Drawing for the job (mm, zero at the part's lowest x, y, z). Coordinates: 2 decimals unless noted, no trailing zeros. Loops run counter-clockwise (first coordinate to the right, second up) from the corner with the lowest first, then second, coordinate; pieces in that order, holes last. Notation, with made-up numbers: (31, -19.5) -> (40, -19.5) arc R26 ccw to (40, 8.5) -> close; hole circle Ø4 at (-22, 87). An arc over 180 degrees is marked (long way). Write each question's results on one line, items separated by ' | '.
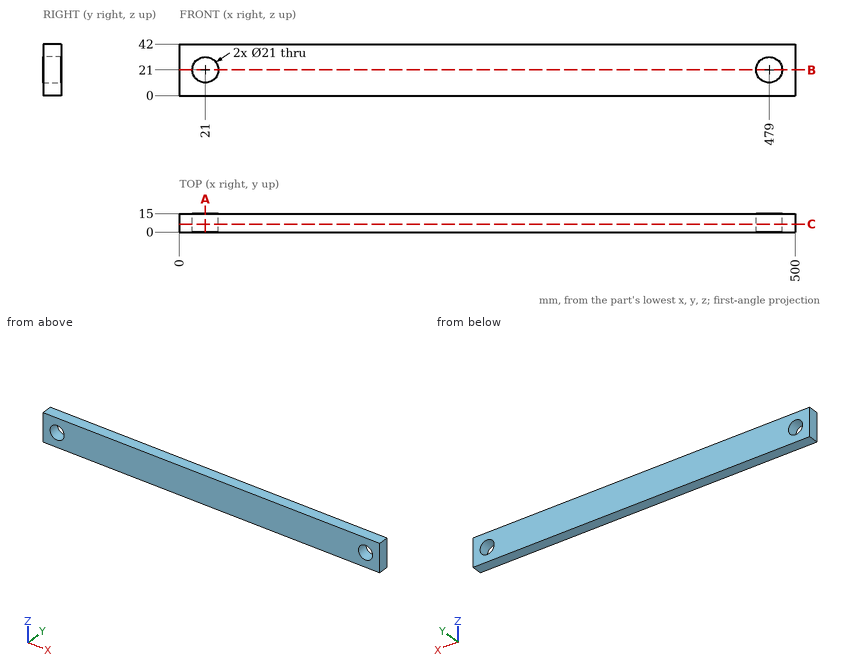
1) Drill centre lines: L1, parallel to X at y = 6.5, z = 23; L2, parallel to Z at x = 479, y = 6.5; L3, parallel to X at y = 4, z = 21. Where is each one in solid material? Low to high. Write a range as from..to.
Outcome:
L1: x = 0..10.69, 31.31..468.69, 489.31..500 | L2: z = 0..10.5, 31.5..42 | L3: x = 0..10.5, 31.5..468.5, 489.5..500
2) Slice it at A-A (x = 21). Write the cut outline in (y, z), then the cut area to 3 significant figures.
Outcome:
outline: (0, 0) -> (15, 0) -> (15, 10.5) -> (0, 10.5) -> close; (0, 31.5) -> (15, 31.5) -> (15, 42) -> (0, 42) -> close | area: 315 mm^2
3) Slice it at B-B (z = 21). Write the cut outline in (x, y), then the cut area to 3 significant figures.
Outcome:
outline: (0, 0) -> (10.5, 0) -> (10.5, 15) -> (0, 15) -> close; (31.5, 0) -> (468.5, 0) -> (468.5, 15) -> (31.5, 15) -> close; (489.5, 0) -> (500, 0) -> (500, 15) -> (489.5, 15) -> close | area: 6,870 mm^2
4) Slice it at C-C (y = 6.5). Write the cut outline in (x, z).
Outcome:
outline: (0, 0) -> (500, 0) -> (500, 42) -> (0, 42) -> close; hole circle Ø21 at (21, 21); hole circle Ø21 at (479, 21)
